Input: part model. Units: mm. Frame: model coordinates. Coordinates: 2 decimals unless noted, no trailing zeros. Loops run counter-clockwise (first coordinate to the right, second up) from the corner with the lowest first, then second, coordinate; pieces in that order, holes last. Notation, with made-up numbers: (-12, 69) -> (33, 69) arc R33 ccw to (33, 107) -> close; hole circle Ø8 at (-16.75, -9.5). An arc over 180 degrees is marked (long way). Answer as a JSON object with one key per item and string values.
from build123d import *

# Parameters (mm, degrees)
SKETCH1_W           = 300
SKETCH1_H           = 20
SKETCH1_W_2         = 10
SKETCH1_H_2         = 10
BOSS_EXTRUDE1_DEPTH = 20
SKETCH6_W           = 10
SKETCH6_H           = 10
CUT_EXTRUDE5_DEPTH  = 10
SKETCH2_W           = 30
SKETCH2_H           = 20
CUT_EXTRUDE1_DEPTH  = 10
SKETCH4_R           = 2.5
CUT_EXTRUDE3_DEPTH  = 153.643375225
CUT_EXTRUDE4_REACH  = 153.658
SKETCH5_R           = 5


with BuildPart() as part:
    # Sketch1 → Boss-Extrude1 (new body)
    with BuildSketch(Plane(origin=(0, 0, 0), x_dir=(1, 0, 0), z_dir=(0, 1, 0))):
        Rectangle(SKETCH1_W, SKETCH1_H)
        with Locations((-145, 15)):
            Rectangle(SKETCH1_W_2, SKETCH1_H_2)
        with Locations((145, 15)):
            Rectangle(SKETCH1_W_2, SKETCH1_H_2)
    extrude(amount=BOSS_EXTRUDE1_DEPTH)

    # Sketch6 → Cut-Extrude5 (cut)
    with BuildSketch(Plane(origin=(0, 0, -20), x_dir=(-1, 0, 0), z_dir=(0, 0, -1))):
        with Locations((-145, 10)):
            Rectangle(SKETCH6_W, SKETCH6_H)
        with Locations((145, 10)):
            Rectangle(SKETCH6_W, SKETCH6_H)
    extrude(amount=-CUT_EXTRUDE5_DEPTH, mode=Mode.SUBTRACT)

    # Sketch2 → Cut-Extrude1 (cut)
    with BuildSketch(Plane(origin=(0, 20, 0), x_dir=(1, 0, 0), z_dir=(0, 1, 0))):
        Rectangle(SKETCH2_W, SKETCH2_H)
    extrude(amount=-CUT_EXTRUDE1_DEPTH, mode=Mode.SUBTRACT)

    # Sketch4 → Cut-Extrude3 (cut, through all)
    with BuildSketch(Plane(origin=(0, 20, 0), x_dir=(1, 0, 0), z_dir=(0, 1, 0))):
        with Locations(Location((-145, 15, 0), (0, 0, 90))):
            Circle(SKETCH4_R)
        with Locations(Location((145, 15, 0), (0, 0, 270))):
            Circle(SKETCH4_R)
    extrude(amount=-CUT_EXTRUDE3_DEPTH, mode=Mode.SUBTRACT)

    # Sketch5 → Cut-Extrude4 (cut, up to next)
    with BuildSketch(Plane(origin=(0, 10, 0), x_dir=(1, 0, 0), z_dir=(0, 1, 0)), mode=Mode.PRIVATE) as cut_extrude4_sk1:
        with Locations(Location((0, 0, 0), (0, 0, 270))):
            Circle(SKETCH5_R)
    cut_extrude4_tool1 = extrude(cut_extrude4_sk1.sketch, amount=-CUT_EXTRUDE4_REACH, mode=Mode.PRIVATE) & part.part
    add(cut_extrude4_tool1.solids().sort_by_distance((0, 10, 0))[0], mode=Mode.SUBTRACT)


solid = part.part
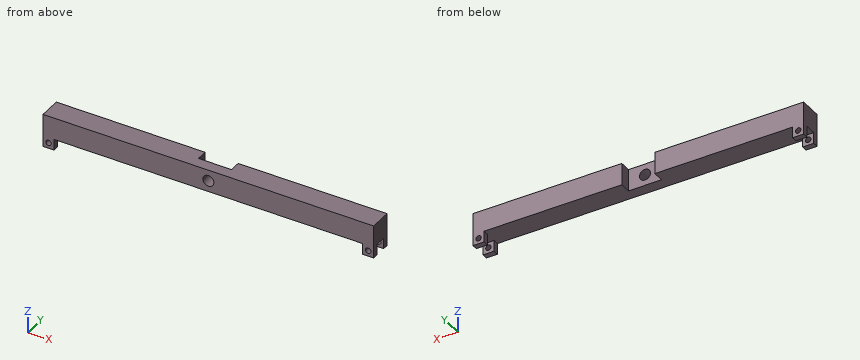
1. Line query: line 1 along X through (y, z) = (17.35, -15); line 2 along Z through (x, y) = (-145, 17); line 3 along X through (y, z) = (10.5, -3.75). Output: solid intervals per line, ascending.
Reply:
{"line 1": "x = -150 to -147.5, -142.5 to -140, 140 to 142.5, 147.5 to 150", "line 2": "z = -20 to -17.5, -12.5 to 10", "line 3": "x = -150 to -15, 15 to 150"}
2. Section query B-B (x = 0). Return loops of the section in (y, z), plus the area to 3 significant figures.
Reply:
{"outline": "(0, -10) -> (10, -10) -> (10, -5) -> (0, -5) -> close; (0, 5) -> (10, 5) -> (10, 10) -> (0, 10) -> close", "area": "100 mm2"}
3. Section query A-A (x = -145). Return loops of the section in (y, z), plus the area to 3 significant figures.
Reply:
{"outline": "(0, -20) -> (5, -20) -> (5, -17.5) -> (0, -17.5) -> close; (0, -12.5) -> (5, -12.5) -> (5, -10) -> (15, -10) -> (15, -12.5) -> (20, -12.5) -> (20, 10) -> (0, 10) -> close; (15, -20) -> (20, -20) -> (20, -17.5) -> (15, -17.5) -> close", "area": "450 mm2"}
4. Section query C-C (z = 0). Return loops of the section in (x, y).
Reply:
{"outline": "(-150, 0) -> (-5, 0) -> (-5, 10) -> (-15, 10) -> (-15, 20) -> (-150, 20) -> close; (5, 0) -> (150, 0) -> (150, 20) -> (15, 20) -> (15, 10) -> (5, 10) -> close"}
5. Section query D-D (y = 2.5). Return loops of the section in (x, z).
Reply:
{"outline": "(-150, -20) -> (-140, -20) -> (-140, -10) -> (140, -10) -> (140, -20) -> (150, -20) -> (150, 10) -> (-150, 10) -> close; hole circle Ø5 at (-145, -15); hole circle Ø10 at (0, 0); hole circle Ø5 at (145, -15)"}
6. Pin query (flat end, axial travel): P1, Ø16, axis at x = 6.5, z = 3.5, coming from the +Y side; P2, Ø10, axis at x = -39, y = 5.5, coming from the -Z side; P3, Ø4.5, axis at x = 145, z = -15, coming from the +Y side. Return the tip coordinate at first contact, or that it passes through.
Reply:
{"P1": "stops at y = 10", "P2": "stops at z = -10", "P3": "passes through"}
